Check sheet for the modelled part. Datum: model origin and axes. Units: mm. Give positions to 0.01 mm unless a question says otherwise; leave off trailing zeros. Loops run counter-clockwise (first coordinate to the right, second up) from the corner with the lowest first, then second, coordinate; pieces in that order, holes last. Notation, with made-up numbers: M 71,15 L 110,15 A8 ccw 110,26 Z; hole C -26,79 d11. An arc over 180 degrees is marked long. Write each question's results on one line, items separated by ' | '. Start each with the question number.
1. Material ranges on line 1 along X through (y, z) = (5.75, 2.15); line 2 along Y through (x, z) = (0, 2.1); line 3 along Y through (x, z) = (0, 2.5), recorded low to high.
2. Sectioned sample at C-C on z = 1.4. Record the cut outline in (x, y), and give its area (3 significant figures).
3. Sectioned sample at A-A on x = 0. Give the number of separate pieces and of enclosed holes in the cut face, and give its area (3 significant figures).
4. Go/stop test with flat-tipped pins: pin 1 (1.5 mm diameter, centred on x = 7.5, z = 1.5, fed in from +Y); pin 2 (1 mm diameter, centred on y = -5.5, z = 0.5, fed in from +X). Record where each tip stops, or that it passes through.
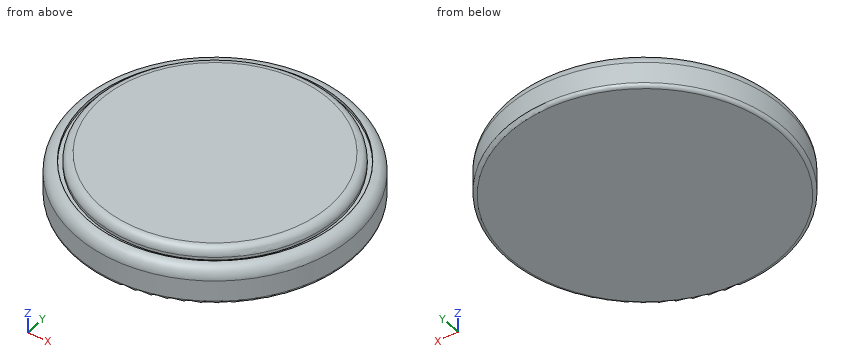
```python
from build123d import *

# Parameters (mm, degrees)
CYLINDER002_R     = 9.16
CYLINDER002_DEPTH = 18
CYLINDER_R        = 10
CYLINDER_DEPTH    = 2.6
CYLINDER001_R     = 8.85
CYLINDER001_DEPTH = 3
FILLET_1_R        = 0.83
FILLET_2_R        = 0.6
FILLET_3_R        = 0.25
CYLINDER003_R     = 9.16
CYLINDER003_DEPTH = 0.2


with BuildPart() as inside_cut:
    # Cylinder002 → Cylinder002 (new body)
    with BuildSketch(Plane.XY.offset(2)):
        Circle(CYLINDER002_R)
    extrude(amount=CYLINDER002_DEPTH)


with BuildPart() as cut:
    # Cylinder → Cylinder (new body)
    with BuildSketch(Plane.XY):
        Circle(CYLINDER_R)
    extrude(amount=CYLINDER_DEPTH)

    # Cut: cut inside_cut
    add(inside_cut.part, mode=Mode.SUBTRACT)


with BuildPart() as battery:
    # Cylinder001 → Cylinder001 (new body)
    with BuildSketch(Plane.XY.offset(0.2)):
        Circle(CYLINDER001_R)
    extrude(amount=CYLINDER001_DEPTH)

    # Fusion: union Cut
    add(cut.part)

    # Fillet 1
    fillet_1_edges = [battery.edges().sort_by_distance(p)[0] for p in [
        (-10, 0, 2.6),
    ]]
    fillet(fillet_1_edges, radius=FILLET_1_R)

    # Fillet 2
    fillet_2_edges = [battery.edges().sort_by_distance(p)[0] for p in [
        (-8.85, 0, 3.2),
    ]]
    fillet(fillet_2_edges, radius=FILLET_2_R)

    # Fillet 3
    fillet_3_edges = [battery.edges().sort_by_distance(p)[0] for p in [
        (-10, 0, 0),
    ]]
    fillet(fillet_3_edges, radius=FILLET_3_R)


with BuildPart() as battery_final:
    # Cylinder003 → Cylinder003 (new body)
    with BuildSketch(Plane.XY.offset(2.2)):
        Circle(CYLINDER003_R)
    extrude(amount=CYLINDER003_DEPTH)

    # Fusion001: union battery
    add(battery.part)


solid = battery_final.part
```
Output values:
1) line 1: -8.07 to -7.13, -6.73 to 6.73, 7.13 to 8.07 | line 2: -9.93 to -9.16, -8.85 to 8.85, 9.16 to 9.93 | line 3: -9.56 to -9.16, -8.85 to 8.85, 9.16 to 9.56
2) outline: C 0,0 d20 | area: 314 mm2
3) separate pieces: 1 | enclosed holes: 2 | area: 61.9 mm2
4) pin 1: y = 7.38 | pin 2: x = 8.66
